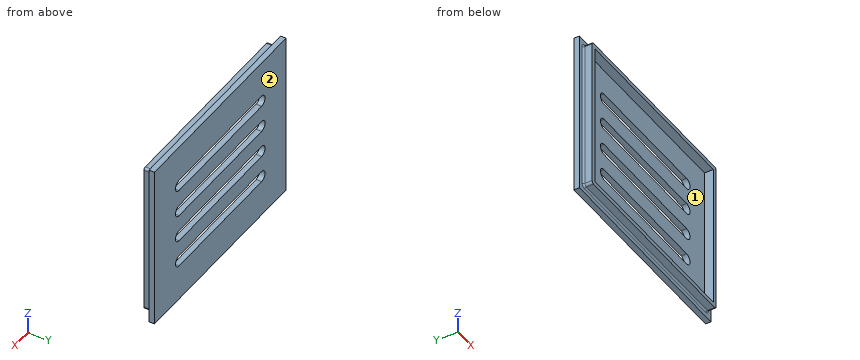
```python
from build123d import *

# Parameters (mm, degrees)
SKETCH1_W           = 90
SKETCH1_H           = 70
SKETCH1_W_2         = 86
SKETCH1_H_2         = 66
EXTRUDE_THIN1_DEPTH = 4
SKETCH2_W           = 95.5
SKETCH2_H           = 75.5
BOSS_EXTRUDE1_DEPTH = 2.5
FILLET1_R           = 1
FILLET2_R           = 0.75


with BuildPart() as part:
    # Sketch1 → Extrude-Thin1 (new body)
    with BuildSketch(Plane(origin=(0, 0, 0), x_dir=(1, 0, 0), z_dir=(0, 1, 0))):
        Rectangle(SKETCH1_W, SKETCH1_H)
        Rectangle(SKETCH1_W_2, SKETCH1_H_2, mode=Mode.SUBTRACT)
    extrude(amount=EXTRUDE_THIN1_DEPTH)

    # Sketch2 → Boss-Extrude1 (add)
    with BuildSketch(Plane(origin=(0, 4, 0), x_dir=(1, 0, 0), z_dir=(0, 1, 0))):
        Rectangle(SKETCH2_W, SKETCH2_H)
        with BuildLine():
            Line((-30, -16.25), (30, -16.25))
            ThreePointArc((30, -16.25), (32.5, -18.75), (30, -21.25))
            Line((30, -21.25), (-30, -21.25))
            ThreePointArc((-30, -21.25), (-32.5, -18.75), (-30, -16.25))
        make_face(mode=Mode.SUBTRACT)
        with BuildLine():
            Line((-30, -3.75), (30, -3.75))
            ThreePointArc((30, -3.75), (32.5, -6.25), (30, -8.75))
            Line((30, -8.75), (-30, -8.75))
            ThreePointArc((-30, -8.75), (-32.5, -6.25), (-30, -3.75))
        make_face(mode=Mode.SUBTRACT)
        with BuildLine():
            Line((-30, 8.75), (30, 8.75))
            ThreePointArc((30, 8.75), (32.5, 6.25), (30, 3.75))
            Line((30, 3.75), (-30, 3.75))
            ThreePointArc((-30, 3.75), (-32.5, 6.25), (-30, 8.75))
        make_face(mode=Mode.SUBTRACT)
        with BuildLine():
            Line((-30, 21.25), (30, 21.25))
            ThreePointArc((30, 21.25), (32.5, 18.75), (30, 16.25))
            Line((30, 16.25), (-30, 16.25))
            ThreePointArc((-30, 16.25), (-32.5, 18.75), (-30, 21.25))
        make_face(mode=Mode.SUBTRACT)
    extrude(amount=BOSS_EXTRUDE1_DEPTH)

    # Fillet1
    fillet1_edges = [part.edges().sort_by_distance(p)[0] for p in [
        (45, 2, 35),
        (-45, 2, 35),
        (-45, 2, -35),
        (45, 2, -35),
    ]]
    fillet(fillet1_edges, radius=FILLET1_R)

    # Fillet2
    fillet2_edges = [part.edges().sort_by_distance(p)[0] for p in [
        (-45, 4, 0),
        (0, 4, -35),
        (45, 4, 0),
        (0, 4, 35),
        (-44.707106781, 4, -34.707106781),
        (44.707106781, 4, -34.707106781),
        (-44.707106781, 4, 34.707106781),
        (44.707106781, 4, 34.707106781),
    ]]
    fillet(fillet2_edges, radius=FILLET2_R)


solid = part.part
```
Geometry check sheet. Reference: the model listing, model coordinates, mm. Face numbers are marked on the shaded views. Give positions to 0.01 mm unless a question says otherwise; leave off trailing zeros. Order: outer loops, then holes, each group sorted by start corner. A loop starts at its lowest first (then second) coordinate and runs counter-clockwise, first axis right, second up. Notation, with made-up numbers: (-10, -38.75) - (13, -38.75) arc R23 ccw to (13, -17.75) - close; hole circle Ø6 at (27, -22.75). An arc over 180 degrees is marked (long way). Write item = value, one per line. Start each with the question number.
1) Section check A-A (y = 1.5). Enter the section's corners in (x, z).
2) Section check D-D (x = -38). Enter the section's corners in (y, z).
3) Scan lines: L1, parallel to Z at x = 20.5, y = 4.75; L2, parallel to Z at x = 39, y = 2; L3, parallel to X at y = 1.75, z = 31. Record each from-to range of solid material in increasing order.
4) Section check B-B (x = 19.5). Count the separate pieces of the cut face and the enclosed holes in it, then the cut area to 3 significant figures.
5) Draft check along X on the marked faces 1 and 2. Enter one of: released by +X, released by -X, zero draft, split by the parting line, or undercut.
6) Section check C-C (z = 18.75). Enter the section's corners in (x, y), then the cut area to 3 significant figures.
7) Gauge pin test, flat ends, axial feed: pin 1 Ø2.5 at (y, z) = (2, -5.5) entering from -X; pin 2 Ø2 at (x, z) = (32.5, 15) entering from -Y; pin 3 Ø1 at (x, y) = (-3.5, 1.5) entering from -Z; pin 4 Ø3 at (x, y) = (-27.5, 3.5) entering from +Z. Record the tip position at first contact, or that the pin passes through.
Geometry check:
q1.outline = (-45, -34) arc R1 ccw to (-44, -35) - (44, -35) arc R1 ccw to (45, -34) - (45, 34) arc R1 ccw to (44, 35) - (-44, 35) arc R1 ccw to (-45, 34) - close; hole (-43, -33) - (43, -33) - (43, 33) - (-43, 33) - close
q2.outline = (0, -35) - (3.25, -35) arc R0.75 cw to (4, -35.75) - (4, -37.75) - (6.5, -37.75) - (6.5, 37.75) - (4, 37.75) - (4, 35.75) arc R0.75 cw to (3.25, 35) - (0, 35) - (0, 33) - (4, 33) - (4, -33) - (0, -33) - close
q3.L1 = -37.75 to -21.25, -16.25 to -8.75, -3.75 to 3.75, 8.75 to 16.25, 21.25 to 37.75
q3.L2 = -35 to -33, 33 to 35
q3.L3 = -45 to -43, 43 to 45
q4.separate_pieces = 5
q4.enclosed_holes = 0
q4.area = 155 mm2
q5.face_1 = undercut
q5.face_2 = zero draft
q6.outline = (-47.75, 4) - (-45.75, 4) arc R0.75 cw to (-45, 3.25) - (-45, 0) - (-43, 0) - (-43, 4) - (-32.5, 4) - (-32.5, 6.5) - (-47.75, 6.5) - close; (32.5, 4) - (43, 4) - (43, 0) - (45, 0) - (45, 3.25) arc R0.75 cw to (45.75, 4) - (47.75, 4) - (47.75, 6.5) - (32.5, 6.5) - close
q6.area = 92.5 mm2
q7.pin_1 = -45
q7.pin_2 = 4
q7.pin_3 = -35
q7.pin_4 = 37.75
